Here's how the part is built. I have some questions about the finished solid (model axes, mm). A direction names the side the tool comes from. Coordinates: 2 decimals unless noted, no trailing zeros. Write each loop counter-clockwise with the first axis right and the second up, starting at its lowest first coordinate (ties: lowest second). Pieces come first, ordered by that corner, then holes.
Item 1: If we mould it in two halves opening along X, with no side actions, what happens to faces 3 (the face through (-1, 0.8, -14)), 4 (the face through (17, 0, -19)), 5 (the face through (47, 0, 41.9))? For each: pulls with the +X half, pulls with the -X half, needs draft (parallel to the pull), parting line crosses it, or undercut.
Item 2: I'm going to push flat-ended pins straight in: P1, Ø0.8, axis at y = 0.5, z = 40, coming from the -X side; P2, Ø0.8, axis at y = 0, z = -48, coming from the +X side; P3, Ø0.5, axis at y = -0.5, z = -49, coming from the -X side. Where does each tip first touch, or does it pass through?
Item 3: I want a section at D-D (x = 40). Please give me the cut outline in (y, z).
Item 4: I want a section at B-B (z = -17). Please give me the cut outline in (x, y).
Item 5: I want a section at C-C (y = 0.4). Count the separate pieces of the cut face and the enclosed holes in it, and give its area (3 significant figures).
Item 6: I want a section at A-A (z = 3). Please give me the cut outline in (x, y), and give its area (3 significant figures).
Item 7: For faces 1 (the face through (-0.05, 0.01, 11.1)), 2 (the face through (-47, 0, 41.9)), which set-ups out of +Z, -Z, +X, -X, +Y, -Y let a thin tool reach every point of the face, with its end or its side?
Item 8: Please list where these lines run through material, in increasing order: line 1 (X direction, y = -0.3, z = 17); line 2 (Z direction, x = -17, y = -0.2); line 3 (X direction, y = 0.05, z = -16).
from build123d import *

# Parameters (mm, degrees)
GENERICCARDPCBDEFINITION_FILLET3_START   = -0.8
GENERICCARDPCBDEFINITION_FILLET3_OUTLI_R = 0.16
GENERICCARDPCBDEFINITION_FILLET3_DEPTH   = 1.6
SKETCH1_R                                = 1
SKETCH1_W                                = 15.4
SKETCH1_H                                = 14.6
SKETCH1_W_2                              = 13.4
SKETCH1_H_2                              = 12.6
CUT_EXTRUDE1_DEPTH                       = 10
F_4_0MM_DOWEL_HOLE1_D                    = 4
F_4_0MM_DOWEL_HOLE1_DEPTH                = 29.81
F_4_0MM_DOWEL_HOLE1_TIP                  = 1.201721238
SKETCH5_R                                = 1.1
CUT_EXTRUDE2_DEPTH                       = 71.516735602
FILLET1_R                                = 0.5


# Read off the part's stored shape, not the designer's step: <GenericCardPCBDefinition>-<Fillet3>
with BuildPart() as part:
    # <GenericCardPCBDefinition>-<Fillet3> outli → <GenericCardPCBDefinition>-<Fillet3> (new body)
    with BuildSketch(Plane(origin=(0, 0, 0), x_dir=(1, 0, 0), z_dir=(0, 1, 0)).offset(GENERICCARDPCBDEFINITION_FILLET3_START)):
        with BuildLine():
            ThreePointArc((-41.232050808, -44.8), (-40.5, -44.067949192), (-39.5, -43.8))
            Line((-39.5, -43.8), (-38.267949192, -43.8))
            ThreePointArc((-38.267949192, -43.8), (-37.914395801, -43.653553391), (-37.767949192, -43.3))
            Line((-37.767949192, -43.3), (-37.767949192, -41.3))
            ThreePointArc((-37.767949192, -41.3), (-37.621502583, -40.946446609), (-37.267949192, -40.8))
            Line((-37.267949192, -40.8), (-35.59, -40.8))
            Line((-35.59, -40.8), (-35.59, -37.1))
            ThreePointArc((-35.59, -37.1), (-35.443553391, -36.746446609), (-35.09, -36.6))
            Line((-35.09, -36.6), (-32.91, -36.6))
            ThreePointArc((-32.91, -36.6), (-32.556446609, -36.746446609), (-32.41, -37.1))
            Line((-32.41, -37.1), (-32.41, -40.8))
            Line((-32.41, -40.8), (-29.59, -40.8))
            Line((-29.59, -40.8), (-29.59, -37.1))
            ThreePointArc((-29.59, -37.1), (-29.443553391, -36.746446609), (-29.09, -36.6))
            Line((-29.09, -36.6), (-26.91, -36.6))
            ThreePointArc((-26.91, -36.6), (-26.556446609, -36.746446609), (-26.41, -37.1))
            Line((-26.41, -37.1), (-26.41, -40.8))
            Line((-26.41, -40.8), (-23.59, -40.8))
            Line((-23.59, -40.8), (-23.59, -37.1))
            ThreePointArc((-23.59, -37.1), (-23.443553391, -36.746446609), (-23.09, -36.6))
            Line((-23.09, -36.6), (-20.91, -36.6))
            ThreePointArc((-20.91, -36.6), (-20.556446609, -36.746446609), (-20.41, -37.1))
            Line((-20.41, -37.1), (-20.41, -40.8))
            Line((-20.41, -40.8), (-18.732050808, -40.8))
            ThreePointArc((-18.732050808, -40.8), (-18.378497417, -40.946446609), (-18.232050808, -41.3))
            Line((-18.232050808, -41.3), (-18.232050808, -43.3))
            ThreePointArc((-18.232050808, -43.3), (-18.085604199, -43.653553391), (-17.732050808, -43.8))
            Line((-17.732050808, -43.8), (-16.5, -43.8))
            ThreePointArc((-16.5, -43.8), (-15.5, -44.067949192), (-14.767949192, -44.8))
            Line((-14.767949192, -44.8), (14.767949192, -44.8))
            ThreePointArc((14.767949192, -44.8), (16.5, -43.8), (18.232050808, -44.8))
            Line((18.232050808, -44.8), (37.767949192, -44.8))
            ThreePointArc((37.767949192, -44.8), (39.5, -43.8), (41.232050808, -44.8))
            Line((41.232050808, -44.8), (44.1, -44.8))
            Line((44.1, -44.8), (49.9, -39))
            Line((49.9, -39), (49.9, 40.7))
            ThreePointArc((49.9, 40.7), (49.753553391, 41.053553391), (49.4, 41.2))
            Line((49.4, 41.2), (47.65, 41.2))
            ThreePointArc((47.65, 41.2), (47.296446609, 41.346446609), (47.15, 41.7))
            Line((47.15, 41.7), (47.15, 46.4))
            ThreePointArc((47.15, 46.4), (47.003553391, 46.753553391), (46.65, 46.9))
            Line((46.65, 46.9), (34.9, 46.9))
            ThreePointArc((34.9, 46.9), (34.546446609, 47.046446609), (34.4, 47.4))
            Line((34.4, 47.4), (34.4, 49.3))
            ThreePointArc((34.4, 49.3), (34.253553391, 49.653553391), (33.9, 49.8))
            Line((33.9, 49.8), (-33.9, 49.8))
            ThreePointArc((-33.9, 49.8), (-34.253553391, 49.653553391), (-34.4, 49.3))
            Line((-34.4, 49.3), (-34.4, 47.4))
            ThreePointArc((-34.4, 47.4), (-34.546446609, 47.046446609), (-34.9, 46.9))
            Line((-34.9, 46.9), (-46.65, 46.9))
            ThreePointArc((-46.65, 46.9), (-47.003553391, 46.753553391), (-47.15, 46.4))
            Line((-47.15, 46.4), (-47.15, 41.7))
            ThreePointArc((-47.15, 41.7), (-47.296446609, 41.346446609), (-47.65, 41.2))
            Line((-47.65, 41.2), (-49.4, 41.2))
            ThreePointArc((-49.4, 41.2), (-49.753553391, 41.053553391), (-49.9, 40.7))
            Line((-49.9, 40.7), (-49.9, -39))
            Line((-49.9, -39), (-44.1, -44.8))
            Line((-44.1, -44.8), (-41.232050808, -44.8))
        make_face()
        with Locations((-35.59, -36.6)):
            Circle(GENERICCARDPCBDEFINITION_FILLET3_OUTLI_R, mode=Mode.SUBTRACT)
        with Locations((-32.41, -36.6)):
            Circle(GENERICCARDPCBDEFINITION_FILLET3_OUTLI_R, mode=Mode.SUBTRACT)
        with Locations((-29.59, -36.6)):
            Circle(GENERICCARDPCBDEFINITION_FILLET3_OUTLI_R, mode=Mode.SUBTRACT)
        with Locations((-26.41, -36.6)):
            Circle(GENERICCARDPCBDEFINITION_FILLET3_OUTLI_R, mode=Mode.SUBTRACT)
        with Locations((-23.59, -36.6)):
            Circle(GENERICCARDPCBDEFINITION_FILLET3_OUTLI_R, mode=Mode.SUBTRACT)
        with Locations((-20.41, -36.6)):
            Circle(GENERICCARDPCBDEFINITION_FILLET3_OUTLI_R, mode=Mode.SUBTRACT)
    extrude(amount=GENERICCARDPCBDEFINITION_FILLET3_DEPTH)

    # Sketch1 → Cut-Extrude1 (cut)
    # profile 1 of 6: a face of its own
    with BuildSketch(Plane(origin=(0, 0.8, 0), x_dir=(1, 0, 0), z_dir=(0, 1, 0))):
        with BuildLine():
            Line((2.3, -7.3), (-2.3, -7.3))
            Line((-2.3, -7.3), (-2.3, -8.8))
            ThreePointArc((-2.3, -8.8), (0, -11.1), (2.3, -8.8))
            Line((2.3, -8.8), (2.3, -7.3))
        make_face()
        with Locations((0, -9)):
            Circle(SKETCH1_R, mode=Mode.SUBTRACT)
    # profile 2 of 6: a face of its own
    with BuildSketch(Plane(origin=(0, 0.8, 0), x_dir=(1, 0, 0), z_dir=(0, 1, 0))):
        Rectangle(SKETCH1_W, SKETCH1_H)
        Rectangle(SKETCH1_W_2, SKETCH1_H_2, mode=Mode.SUBTRACT)
    # profile 3 of 6: a face of its own
    with BuildSketch(Plane(origin=(0, 0.8, 0), x_dir=(1, 0, 0), z_dir=(0, 1, 0))):
        Rectangle(SKETCH1_W_2, SKETCH1_H_2)
    # profile 4 of 6: a face of its own
    with BuildSketch(Plane(origin=(0, 0.8, 0), x_dir=(1, 0, 0), z_dir=(0, 1, 0))):
        with BuildLine():
            Line((-2.3, 8.8), (-2.3, 7.3))
            Line((-2.3, 7.3), (2.3, 7.3))
            Line((2.3, 7.3), (2.3, 8.8))
            ThreePointArc((2.3, 8.8), (0, 11.1), (-2.3, 8.8))
        make_face()
        with Locations((0, 9)):
            Circle(SKETCH1_R, mode=Mode.SUBTRACT)
    # profile 5 of 6: a face of its own
    with BuildSketch(Plane(origin=(0, 0.8, 0), x_dir=(1, 0, 0), z_dir=(0, 1, 0))):
        with Locations((0, 9)):
            Circle(SKETCH1_R)
    # profile 6 of 6: a face of its own
    with BuildSketch(Plane(origin=(0, 0.8, 0), x_dir=(1, 0, 0), z_dir=(0, 1, 0))):
        with Locations((0, -9)):
            Circle(SKETCH1_R)
    extrude(amount=-CUT_EXTRUDE1_DEPTH, mode=Mode.SUBTRACT)

    # Ø4.0mm Dowel Hole1
    with Locations(Plane(origin=(0, -0.8, 0), x_dir=(-1, 0, 0), z_dir=(0, -1, 0))):
        with Locations((17, -17), (-17, -17), (17, 17), (-17, 17)):
            Hole(F_4_0MM_DOWEL_HOLE1_D / 2, depth=F_4_0MM_DOWEL_HOLE1_DEPTH)
            with Locations((0, 0, -(F_4_0MM_DOWEL_HOLE1_DEPTH + F_4_0MM_DOWEL_HOLE1_TIP / 2))):  # 118° drill point
                Cone(0, F_4_0MM_DOWEL_HOLE1_D / 2, F_4_0MM_DOWEL_HOLE1_TIP, mode=Mode.SUBTRACT)

    # Sketch5 → Cut-Extrude2 (cut, through all)
    with BuildSketch(Plane.XZ.offset(0.8)):
        with Locations(Location((-33.8, -30.4, 0), (0, 0, 270))):
            Circle(SKETCH5_R)
        with Locations(Location((-21.8, -30.4, 0), (0, 0, 270))):
            Circle(SKETCH5_R)
        with Locations(Location((-21.8, -0.4, 0), (0, 0, 270))):
            Circle(SKETCH5_R)
    extrude(amount=-CUT_EXTRUDE2_DEPTH, mode=Mode.SUBTRACT)

    # Fillet1
    fillet1_edges = [part.edges().sort_by_distance(p)[0] for p in [
        (-2.3, 0, 7.3),
        (-2.3, 0, -7.3),
        (2.3, 0, -7.3),
        (2.3, 0, 7.3),
    ]]
    fillet(fillet1_edges, radius=FILLET1_R)


solid = part.part
Answer:
1. face 3: needs draft
1. face 4: undercut
1. face 5: pulls with the +X half
2. P1: stops at x = -49.3
2. P2: stops at x = 34.4
2. P3: stops at x = -34.4
3. outline: (-0.8, -46.9) - (0.8, -46.9) - (0.8, 43.86) - (-0.8, 43.86) - close
4. outline: (-49.9, -0.8) - (-19, -0.8) - (-19, 0.8) - (-49.9, 0.8) - close; (-15, -0.8) - (15, -0.8) - (15, 0.8) - (-15, 0.8) - close; (19, -0.8) - (49.9, -0.8) - (49.9, 0.8) - (19, 0.8) - close
5. separate pieces: 1
5. enclosed holes: 14
5. area: 8,840 mm2
6. outline: (-49.9, -0.8) - (-7.7, -0.8) - (-7.7, 0.8) - (-49.9, 0.8) - close; (7.7, -0.8) - (49.9, -0.8) - (49.9, 0.8) - (7.7, 0.8) - close
6. area: 135 mm2
7. face 1: +Y, -Y
7. face 2: +Z, -X, +Y, -Y
8. line 1: x = -49.9 to -19, -15 to 15, 19 to 49.9
8. line 2: z = -49.8 to -19, -15 to 15, 19 to 43.8
8. line 3: x = -49.9 to -18.73, -15.27 to 15.27, 18.73 to 49.9
